Build history of the part. All positions in model axes, mm. A direction names the side the tool comes from. Give positions to 0.01 mm unless a question says otherwise; leave off trailing zeros. Order: outer loops, then holes, each group sorted by start corner. A loop starts at its lowest first (then second) coordinate and runs counter-clockwise, first axis right, second up. Notation, with made-up numbers: (-24.75, 16.5) -> (-14.75, 16.5) arc R24 ccw to (-14.75, 54.5) -> close; hole circle Ø4 at (54, -19). An arc over 180 degrees is marked (long way). One line per item, written item: value. Start each with the question number.
(1) Saw through at D-D on x = 300. Give the cut face in (y, z), plus the area to 3 significant figures.
(2) Pin check, flat tips, straight feed: pin 1 (10 mm diameter, centred on x = 274, y = 32, fed in from -Z); pin 2 (10 mm diameter, centred on y = 33.5, z = -68, fed in from -X); pin 3 (6 mm diameter, centred on y = 31.5, z = -59, fed in from +X); pin 4 (10 mm diameter, centred on x = 285, y = 31, fed in from -Z). Stop position of each tip, or through.
(3) Saw through at B-B on y = 35. Give the cut face in (x, z).
(4) Saw through at A-A on x = 271. Give the cut face in (y, z), plus the area to 3 significant figures.
(5) Saw through at C-C on y = 31.5. Give the cut face in (x, z).
(6) Probe line 1 (Y direction, x = 271, z = -51.3); line 2 (X direction, y = 35, z = -51.05); line 3 (Z direction, x = 303, y = 33). List the from-to ranges inside material, lowest first.
(7) Which spindle directions (+Z, -Z, +X, -X, +Y, -Y) get a long thin tool onto all of the face, cutting with end or side? Do faces 1 (the flat face through (287, 30, -63)), 2 (the flat face through (288, 30, -62)), 3 (the cylindrical face through (279.4, 23.8, -51)). Say none if no direction does.
(8) Two-plate mould, pull along Y, no slides. Class faces 4 (the flat face through (267, 30, -51)), 5 (the cylindrical face through (279.4, 33.8, -51)): +Y half, -Y half, draft (parallel to the pull), parting line (faces both ways), or undercut.
```python
from build123d import *

# Parameters (mm, degrees)
CYLINDER003_R     = 2
CYLINDER003_DEPTH = 10
BOX003_W          = 25
BOX003_H          = 20
BOX003_DEPTH      = 1
BOX002_W          = 20
BOX002_H          = 1
BOX002_DEPTH      = 23
BOX004_W          = 20
BOX004_H          = 20
BOX004_DEPTH      = 2


with BuildPart() as cylinder003:
    # Cylinder003 → Cylinder003 (new body)
    with BuildSketch(Plane(origin=(-7, 5, 20), x_dir=(1, 0, 0), z_dir=(0, 0, 1))):
        Circle(CYLINDER003_R)
    extrude(amount=CYLINDER003_DEPTH)


with BuildPart() as cylinder004:
    # Link base: copy of Cylinder003
    add(cylinder003.part)


with BuildPart() as cylinder004_1:
    # Link placement: moved
    add(cylinder004.part.moved(Location((-10, 0, 0))))


with BuildPart() as cylinder005:
    # Link001 base: copy of Cylinder003
    add(cylinder003.part)


with BuildPart() as cylinder005_1:
    # Link001 placement: moved
    add(cylinder005.part.moved(Location((-10, 10, 0))))


with BuildPart() as cylinder006:
    # Link002 base: copy of Cylinder003
    add(cylinder003.part)


with BuildPart() as cylinder006_1:
    # Link002 placement: moved
    add(cylinder006.part.moved(Location((0, 10, 0))))


with BuildPart() as fusion004:
    # Fusion004 base: copy of Cylinder003
    add(cylinder003.part)

    # Fusion004: union Cylinder004, Cylinder005, Cylinder006
    add(cylinder004_1.part)
    add(cylinder005_1.part)
    add(cylinder006_1.part)


with BuildPart() as s_abajo:
    # Box003 → Box003 (new body)
    with BuildSketch(Plane(origin=(287, 20, -74), x_dir=(1, 0, 0), z_dir=(0, 0, 1))):
        with Locations((12.5, 10)):
            Rectangle(BOX003_W, BOX003_H)
    extrude(amount=BOX003_DEPTH)


with BuildPart() as s_lateral:
    # Box002 → Box002 (new body)
    with BuildSketch(Plane(origin=(288, 20, -73), x_dir=(0, 1, 0), z_dir=(0, 0, 1))):
        with Locations((10, 0.5)):
            Rectangle(BOX002_W, BOX002_H)
    extrude(amount=BOX002_DEPTH)


with BuildPart() as soporte:
    # Box004 → Box004 (new body)
    with BuildSketch(Plane(origin=(267, 20, -52), x_dir=(1, 0, 0), z_dir=(0, 0, 1))):
        with Locations((10, 10)):
            Rectangle(BOX004_W, BOX004_H)
    extrude(amount=BOX004_DEPTH)

    # Fusion003: union s_abajo, s_lateral
    add(s_abajo.part)
    add(s_lateral.part)


with BuildPart() as soporte_1:
    # Fusion003 placement: moved
    add(soporte.part.moved(Location((-288, -20, 73))))

    # Cut001: cut Fusion004
    add(fusion004.part, mode=Mode.SUBTRACT)


with BuildPart() as soporte_2:
    # Cut001 placement: moved
    add(soporte_1.part.moved(Location((288, 20, -73))))


solid = soporte_2.part
```
Results below:
1. outline: (20, -74) -> (40, -74) -> (40, -73) -> (20, -73) -> close
1. area: 20.0 mm²
2. pin 1: stops at z = -52
2. pin 2: stops at x = 287
2. pin 3: stops at x = 288
2. pin 4: stops at z = -74
3. outline: (267, -52) -> (269, -52) -> (269, -50) -> (267, -50) -> close; (273, -52) -> (279, -52) -> (279, -50) -> (273, -50) -> close; (283, -52) -> (287, -52) -> (287, -74) -> (312, -74) -> (312, -73) -> (288, -73) -> (288, -50) -> (283, -50) -> close
4. outline: (20, -52) -> (23, -52) -> (23, -50) -> (20, -50) -> close; (27, -52) -> (33, -52) -> (33, -50) -> (27, -50) -> close; (37, -52) -> (40, -52) -> (40, -50) -> (37, -50) -> close
4. area: 24.0 mm²
5. outline: (267, -52) -> (287, -52) -> (287, -74) -> (312, -74) -> (312, -73) -> (288, -73) -> (288, -50) -> (267, -50) -> close
6. line 1: y = 20 to 23, 27 to 33, 37 to 40
6. line 2: x = 267 to 269, 273 to 279, 283 to 288
6. line 3: z = -74 to -73
7. face 1: -Z, -X, +Y, -Y
7. face 2: +Z, +X, +Y, -Y
7. face 3: +Z, -Z
8. face 4: draft
8. face 5: undercut
